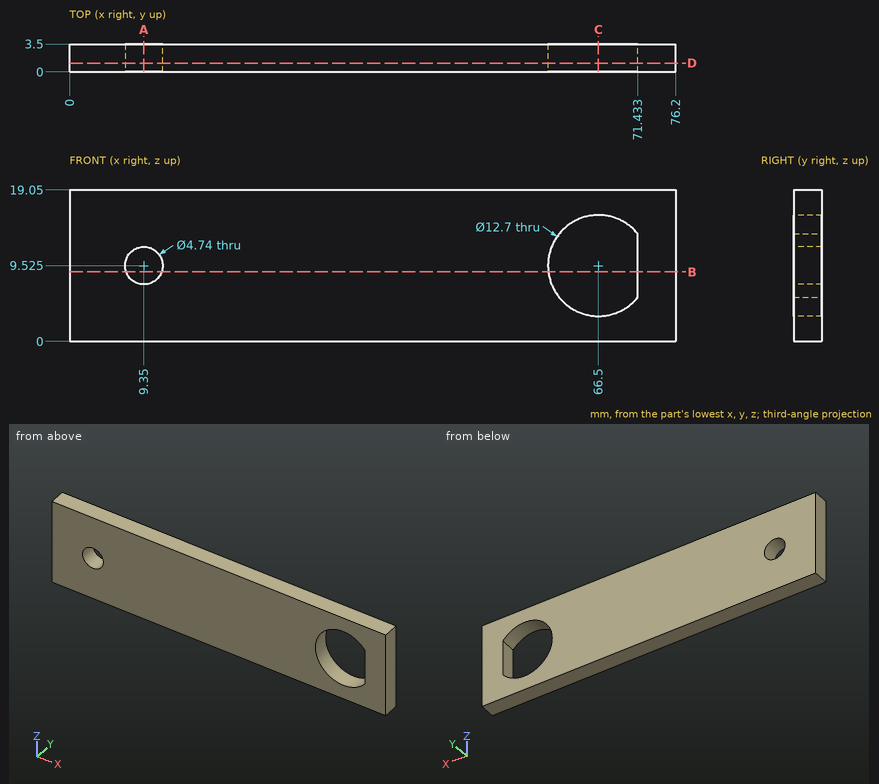
Check sheet for the drawn part. Datum: minimum x, y, z corner. Units: mm. Give positions to 0.01 mm unless a question says otherwise; leave off trailing zeros. Write each loop counter-clockwise with the first axis right and the second up, starting at its lowest first coordinate (ties: lowest second). Pieces come first, ordered by that corner, then holes.
(1) Material ranges on line 1 (Z direction, x = 66.5, y = 1.3) (3 decimals); line 2 (X direction, y = 2.55, z = 9.25); line 3 (Z direction, x = 9.35, y = 0.9) (3 decimals), recorded low to high.
(2) Cross-section at C-C (x = 66.5). Enter the section's corners in (y, z) (3 decimals).
(3) Cross-section at A-A (x = 9.35). Enter the section's corners in (y, z) (3 decimals).
(4) Cross-section at D-D (y = 1.1). State how many separate pieces and enclosed holes the cut face has, plus the area to 3 significant figures.
(5) Gauge pin test, flat end, axial feed: pin 1 (7.5 mm diameter, centred on x = 66.5, z = 9.525, fed in from -Y). Record the tip position at first contact, or that the pin passes through.
(6) Cross-section at B-B (z = 8.75). Enter the section's corners in (x, y), plus the area to 3 significant figures.
Worked out:
1. line 1: z = 0 to 3.175, 15.875 to 19.05
1. line 2: x = 0 to 7, 11.7 to 60.16, 71.43 to 76.2
1. line 3: z = 0 to 7.155, 11.895 to 19.05
2. outline: (0, 0) - (3.5, 0) - (3.5, 3.175) - (0, 3.175) - close; (0, 15.875) - (3.5, 15.875) - (3.5, 19.05) - (0, 19.05) - close
3. outline: (0, 0) - (3.5, 0) - (3.5, 7.155) - (0, 7.155) - close; (0, 11.895) - (3.5, 11.895) - (3.5, 19.05) - (0, 19.05) - close
4. separate pieces: 1
4. enclosed holes: 2
4. area: 1,320 mm2
5. pin 1: passes through
6. outline: (0, 0) - (7.11, 0) - (7.11, 3.5) - (0, 3.5) - close; (11.59, 0) - (60.2, 0) - (60.2, 3.5) - (11.59, 3.5) - close; (71.43, 0) - (76.2, 0) - (76.2, 3.5) - (71.43, 3.5) - close
6. area: 212 mm2
